Verification items for this drawing (mm, ordinates from the low corner). A direction names the side the tool comes from. Round coordinates to 2 decimals unless told otherwise and drop trailing zeros. Order: outer loops, then holes, each group sorted by start corner. A loop starts at its lowest first (then second) coordinate and runs counter-clockwise, first axis right, second up. Notation, with made-up numbers: M 62.25,-3.75 L 67.25,-3.75 A32 cw 67.25,33.25 Z; hole C -7,-5.75 d1. An arc over 180 degrees is marked long. Return JSON: item names as keys, results as strings. Group by question number.
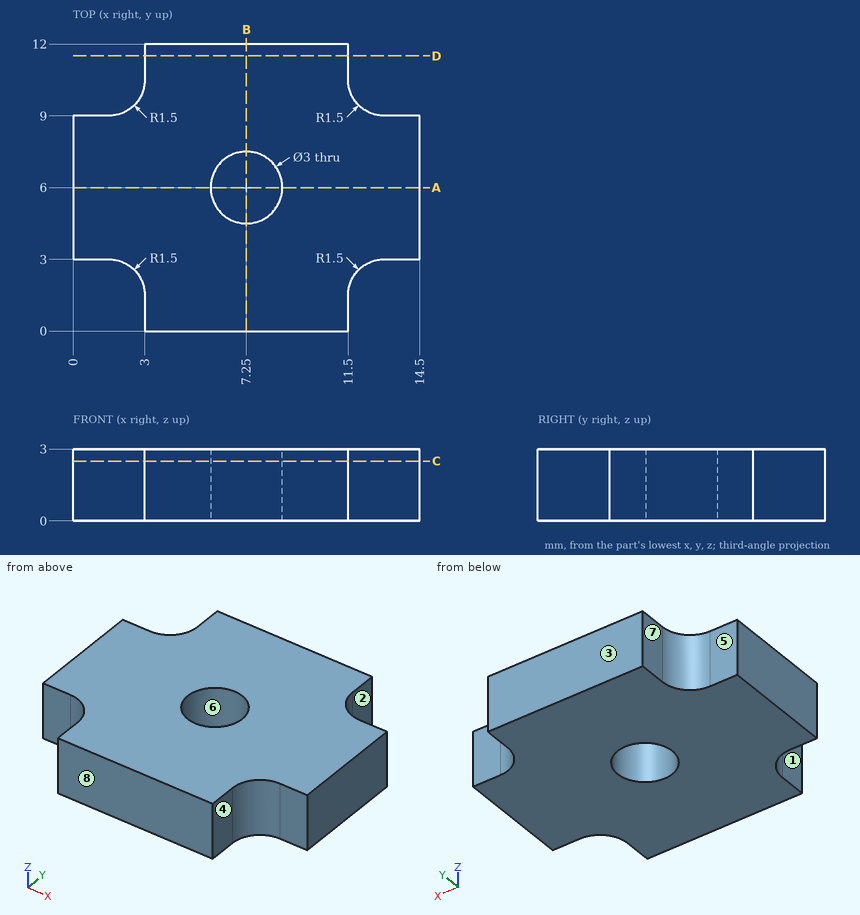
1. Cross-section at C-C (z = 2.5). Enter the section's corners in (x, y).
2. Cross-section at B-B (x = 7.25). Enter the section's corners in (y, z), plus the area to 3 significant figures.
3. Draft check along X on the marked faces 6, 7 and 8. Enter one of: +X half, -X half, draft (parallel to the pull), parting line (faces both ways), or undercut.
4. Cross-section at A-A (y = 6). Enter the section's corners in (x, z), plus the area to 3 significant figures.
5. Go/stop test with flat-tipped pins: pin 1 (5 mm diameter, centred on x = 7.25, y = 6, fed in from +Z); pin 2 (1.6 mm diameter, centred on y = 11.5, z = 1, fed in from +X); pin 3 (1.2 mm diameter, centred on x = 13.5, z = 2, fed in from +Y); pin 4 (1.6 mm diameter, centred on y = 11.5, z = 1, fed in from -X). Record where each tip stops, or that it passes through.
6. Access from +Z, -Z, +X, -X, +Y, -Y to the whole of each face (thin tool, end or side, straight path). Record for the marked faces 1, 2, 3, 4 and 5.
7. Thickness scan on line 1 along Y through (x, z) = (7.25, 2); line 2 along X through (y, z) = (6, 1.05); line 3 along X through (y, z) = (0.5, 1.95). Record the ranges inside material, lowest first. Write a range as from..to.
8. Cross-section at D-D (y = 11.5). Enter the section's corners in (x, z).
Computed:
{
 "1": {"outline": "M 0,3 L 1.5,3 A1.5 cw 3,1.5 L 3,0 L 11.5,0 L 11.5,1.5 A1.5 cw 13,3 L 14.5,3 L 14.5,9 L 13,9 A1.5 cw 11.5,10.5 L 11.5,12 L 3,12 L 3,10.5 A1.5 cw 1.5,9 L 0,9 Z; hole C 7.25,6 d3"},
 "2": {"outline": "M 0,0 L 4.5,0 L 4.5,3 L 0,3 Z; M 7.5,0 L 12,0 L 12,3 L 7.5,3 Z", "area": "27.0 mm²"},
 "3": {"face 6": "undercut", "face 7": "-X half", "face 8": "draft"},
 "4": {"outline": "M 0,0 L 5.75,0 L 5.75,3 L 0,3 Z; M 8.75,0 L 14.5,0 L 14.5,3 L 8.75,3 Z", "area": "34.5 mm²"},
 "5": {"pin 1": "stops at z = 3", "pin 2": "stops at x = 11.5", "pin 3": "stops at y = 9", "pin 4": "stops at x = 3"},
 "6": {"face 1": "+Z, -Z, -X, -Y", "face 2": "+Z, -Z, +X, +Y", "face 3": "+Z, -Z, +X, -X, +Y", "face 4": "+Z, -Z, +X, -Y", "face 5": "+Z, -Z, -X, +Y"},
 "7": {"line 1": "y = 0..4.5, 7.5..12", "line 2": "x = 0..5.75, 8.75..14.5", "line 3": "x = 3..11.5"},
 "8": {"outline": "M 3,0 L 11.5,0 L 11.5,3 L 3,3 Z"}
}
